```python
from build123d import *

# Parameters (mm, degrees)
BOSS_EXTRUDE1_DEPTH = 1219.2
CHAMFER1_SIZE       = 25.4


with BuildPart() as part:
    # Sketch1 → Boss-Extrude1 (new body)
    with BuildSketch(Plane.XY):
        Polygon((0, 0), (0, -25.4), (-6.35, -25.4), (-6.35, -6.35), (-25.4, -6.35), (-25.4, 0), align=None)
    extrude(amount=BOSS_EXTRUDE1_DEPTH)

    # Chamfer1
    chamfer1_edges = [part.edges().sort_by_distance(p)[0] for p in [
        (-25.4, -3.175, 0),
        (-25.4, -3.175, 1219.2),
    ]]
    chamfer(chamfer1_edges, length=CHAMFER1_SIZE - 0.0001)  # a hair under: the kernel refuses the full size


solid = part.part
```
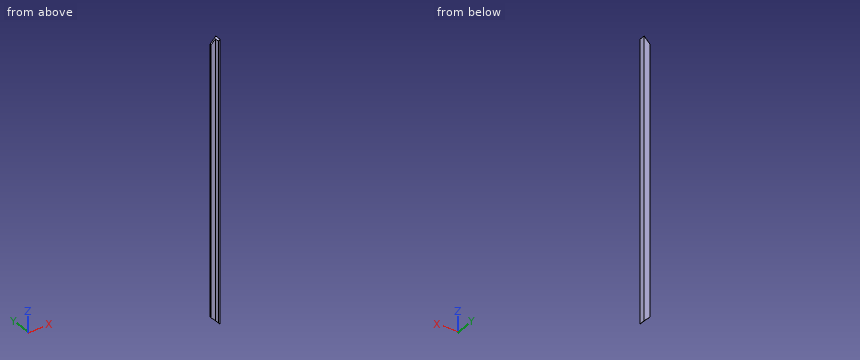
Design review of the part built by this model. Coordinates are the model's own, in mm. Give positions to 0.01 mm unless a question says otherwise; leave off trailing zeros. Loops run counter-clockwise (first coordinate to the right, second up) from the corner with the lowest first, then second, coordinate; pieces in that order, holes last. Notation, with made-up numbers: (35.25, 34) -> (70.25, 34) arc R19 ccw to (70.25, 48) -> close; hole circle Ø4 at (14.5, 22). An arc over 180 degrees is marked (long way). Write each question's results on one line, items separated by ' | '.
Q1. Wall thickness on L1, parallel to Y at x = -13.25, z = 500.5; L2, parallel to Z at x = -24.5, y = -3: over which ranges is each line inside the solid? List them lowest first.
Reply:
L1: y = -6.35 to 0 | L2: z = 24.5 to 1194.7
Q2. Take a section at C-C, the plane x = -21. Write out the cut boundary in (y, z), plus the area to 3 significant figures.
Reply:
outline: (-6.35, 21) -> (0, 21) -> (0, 1198.2) -> (-6.35, 1198.2) -> close | area: 7,480 mm²
Q3. For pin 1 Ø5 at (x, z) = (-8, 452.5) entering from -Y; pin 2 Ø1.5 at (x, y) = (-21.5, -4) entering from +Z; pin 3 Ø12 at (x, y) = (-8, -17) entering from +Z; pin 4 Ø5.5 at (y, z) = (-17.5, 473) entering from -X, all flat-tipped, find the tip position at first contact; note any pin that passes through.
Reply:
pin 1: stops at y = -25.4 | pin 2: stops at z = 1198.45 | pin 3: stops at z = 1217.2 | pin 4: stops at x = -6.35
Q4. Take a section at B-B, the plane z = 1095. Write out the cut boundary in (x, y).
Reply:
outline: (-25.4, -6.35) -> (-6.35, -6.35) -> (-6.35, -25.4) -> (0, -25.4) -> (0, 0) -> (-25.4, 0) -> close
